Part model, mm, in its own coordinate system. A direction names the side the tool comes from. Round coordinates to 2 decimals unless told otherwise and drop trailing zeros. Loops run counter-clockwise (first coordinate to the right, second up) from the corner with the lowest first, then second, coordinate; pieces in that order, holes last.
from build123d import *

# Parameters (mm, degrees)
BOSS_EXTRUDE1_DEPTH = 6.35
SKETCH3_R           = 1.225
CUT_EXTRUDE1_DEPTH  = 317.295028415


with BuildPart() as part:
    # Sketch2 → Boss-Extrude1 (new body)
    with BuildSketch(Plane(origin=(0, 0, 0), x_dir=(1, 0, 0), z_dir=(0, 1, 0))):
        Polygon((0, 0), (266.65, 0), (266.65, 100), (237.633187959, 107.617389248), (231.996319915, 86.144948337), (220.389595099, 89.191904036), (226.026463142, 110.664344947), (212.485284189, 114.219126596), (209.94615444, 104.546855915), (199.94615444, 107.172019988), (202.485284189, 116.844290668), (0, 170), align=None)
    extrude(amount=BOSS_EXTRUDE1_DEPTH)

    # Sketch3 → Cut-Extrude1 (cut, through all)
    with BuildSketch(Plane(origin=(0, 6.35, 0), x_dir=(1, 0, 0), z_dir=(0, 1, 0))):
        with Locations(Location((15, 150.554003041, 0), (0, 0, 270))):
            Circle(SKETCH3_R)
        with Locations(Location((15, 15, 0), (0, 0, 270))):
            Circle(SKETCH3_R)
        with Locations(Location((251.65, 15, 0), (0, 0, 270))):
            Circle(SKETCH3_R)
    extrude(amount=-CUT_EXTRUDE1_DEPTH, mode=Mode.SUBTRACT)


solid = part.part
1) Slice it at A-A, the plane y = 4. Give the cut face in (x, z) (3 decimals), then the cut area to 3 significant figures.
Values:
outline: (0, -170) - (202.485, -116.844) - (199.946, -107.172) - (209.946, -104.547) - (212.485, -114.219) - (226.026, -110.664) - (220.39, -89.192) - (231.996, -86.145) - (237.633, -107.617) - (266.65, -100) - (266.65, 0) - (0, 0) - close; hole circle Ø2.45 at (15, -150.554); hole circle Ø2.45 at (15, -15); hole circle Ø2.45 at (251.65, -15)
area: 35,600 mm2
2) Slice it at B-B, the plane x = 191.5. Give the cut face in (y, z), then the cut area to 3 significant figures.
Values:
outline: (0, -119.73) - (6.35, -119.73) - (6.35, 0) - (0, 0) - close
area: 760 mm2
3) Mould opens along Z. For faces 1 (the face through (205.02, 3.13, -105.84)), 2 (the face through (211.233, 3.131, -109.451)), 3 (the face through (0, 3, -86)), 4 (the face through (131, 3, 0)) say: released by +Z, released by -Z, zero draft, split by the parting line, or undercut.
Values:
face 1: undercut
face 2: released by -Z
face 3: zero draft
face 4: released by +Z
4) Tool access for faces 5 (the face through (234.854, 3.131, -97.031)), 6 (the face through (102.66, 3.13, -143.05)), 7 (the face through (226.27, 3.13, -87.65)): list every direction of +Z, -Z, +X, -X, +Y, -Y with a clear straight run to the whole face (end or side of a thin tool).
Values:
face 5: -Z, +Y, -Y
face 6: -Z, +X, +Y, -Y
face 7: +Y, -Y
5) Slice it at C-C, the plane x = 97. Give the cut face in (y, z).
Values:
outline: (0, -144.54) - (6.35, -144.54) - (6.35, 0) - (0, 0) - close
6) Wall check: line 1 along X through (y, z) = (3, -15) (3 decimals); line 2 along Z through (x, y) = (162.5, 4.75); line 3 along X through (y, z) = (4.25, -95.5). Give the ranges that are in metal, low to high.
Values:
line 1: x = 0 to 13.775, 16.225 to 250.425, 252.875 to 266.65
line 2: z = -127.34 to 0
line 3: x = 0 to 222.05, 234.45 to 266.65
7) Drop flat-ended pins along their axis: pin 1 Ø1 at (x, z) = (142.5, -113.5) entering from -Y; pin 2 Ø1.5 at (y, z) = (3, -115) entering from +X. Give the stop position or say it passes through.
Values:
pin 1: stops at y = 0
pin 2: stops at x = 202.2
